Check sheet for the modelled part. Datum: model origin and axes. Units: mm. Round coordinates to 2 decimals unless told otherwise and drop trailing zeros. Loops run counter-clockwise (first coordinate to the right, second up) from the corner with the lowest first, then second, coordinate; pieces in that order, holes last. Notation, with made-up numbers: (69.25, -1.75) - (115.25, -1.75) arc R25 ccw to (115.25, 20.25) - close; hole circle Ø11 at (23.5, 8.25). An arc over 180 degrees is marked (long way). Put each result on its own line as item: value. Start each with the question number.
Item 1: Section check D-D, the plane x = 10.5. Record the cut outline in (y, z) (3 decimals), and give its area (3 significant figures).
Item 2: Material ranges on line 1 along X through (y, z) = (2.9, -32); line 2 along Z through (x, y) = (41, 0.5); line 3 along X through (y, z) = (1.55, 0), recorded low to high.
Item 3: Section check A-A, the plane x = -38.5. Record the cut outline in (y, z) (3 decimals).
Item 4: Section check C-C, the plane z = 0. Record the cut outline in (x, y) (3 decimals).
Item 5: Section check B-B, the plane y = 1. Record the cut outline in (x, z).
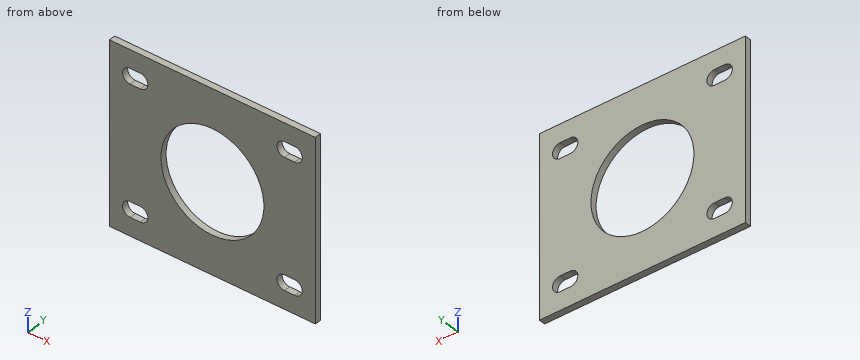
from build123d import *

# Parameters (mm, degrees)
SKETCH1_W           = 101.6
SKETCH1_H           = 88.9
SKETCH1_R           = 25.4
BOSS_EXTRUDE1_DEPTH = 3.175
CUT_EXTRUDE1_DEPTH  = 68.576054376


with BuildPart() as part:
    # Sketch1 → Boss-Extrude1 (new body)
    with BuildSketch(Plane(origin=(0, 0, 0), x_dir=(1, 0, 0), z_dir=(0, 1, 0))):
        Rectangle(SKETCH1_W, SKETCH1_H)
        with Locations(Location((0, 0, 0), (0, 0, 270))):
            Circle(SKETCH1_R, mode=Mode.SUBTRACT)
    extrude(amount=BOSS_EXTRUDE1_DEPTH)

    # Sketch2 → Cut-Extrude1 (cut, through all)
    with BuildSketch(Plane(origin=(0, 3.175, 0), x_dir=(1, 0, 0), z_dir=(0, 1, 0))):
        with BuildLine():
            Line((-40.6, 35.5), (-35.6, 35.5))
            ThreePointArc((-35.6, 35.5), (-31.85, 31.75), (-35.6, 28))
            Line((-35.6, 28), (-40.6, 28))
            ThreePointArc((-40.6, 28), (-44.35, 31.75), (-40.6, 35.5))
        make_face()
        with BuildLine():
            Line((-40.6, -28), (-35.6, -28))
            ThreePointArc((-35.6, -28), (-31.85, -31.75), (-35.6, -35.5))
            Line((-35.6, -35.5), (-40.6, -35.5))
            ThreePointArc((-40.6, -35.5), (-44.35, -31.75), (-40.6, -28))
        make_face()
        with BuildLine():
            Line((35.6, 35.5), (40.6, 35.5))
            ThreePointArc((40.6, 35.5), (44.35, 31.75), (40.6, 28))
            Line((40.6, 28), (35.6, 28))
            ThreePointArc((35.6, 28), (31.85, 31.75), (35.6, 35.5))
        make_face()
        with BuildLine():
            Line((35.6, -28), (40.6, -28))
            ThreePointArc((40.6, -28), (44.35, -31.75), (40.6, -35.5))
            Line((40.6, -35.5), (35.6, -35.5))
            ThreePointArc((35.6, -35.5), (31.85, -31.75), (35.6, -28))
        make_face()
    extrude(amount=-CUT_EXTRUDE1_DEPTH, mode=Mode.SUBTRACT)


solid = part.part
Check result:
1. outline: (0, -44.45) - (3.175, -44.45) - (3.175, -23.128) - (0, -23.128) - close; (0, 23.128) - (3.175, 23.128) - (3.175, 44.45) - (0, 44.45) - close
1. area: 135 mm²
2. line 1: -50.8 to -44.34, -31.86 to 31.86, 44.34 to 50.8
2. line 2: -44.45 to -35.48, -28.02 to 28.02, 35.48 to 44.45
2. line 3: -50.8 to -25.4, 25.4 to 50.8
3. outline: (0, -44.45) - (3.175, -44.45) - (3.175, -35.5) - (0, -35.5) - close; (0, -28) - (3.175, -28) - (3.175, 28) - (0, 28) - close; (0, 35.5) - (3.175, 35.5) - (3.175, 44.45) - (0, 44.45) - close
4. outline: (-50.8, 0) - (-25.4, 0) - (-25.4, 3.175) - (-50.8, 3.175) - close; (25.4, 0) - (50.8, 0) - (50.8, 3.175) - (25.4, 3.175) - close
5. outline: (-50.8, -44.45) - (50.8, -44.45) - (50.8, 44.45) - (-50.8, 44.45) - close; hole (-40.6, -35.5) - (-35.6, -35.5) arc R3.75 ccw to (-35.6, -28) - (-40.6, -28) arc R3.75 ccw to start; hole (-40.6, 28) - (-35.6, 28) arc R3.75 ccw to (-35.6, 35.5) - (-40.6, 35.5) arc R3.75 ccw to start; hole circle Ø50.8 at (0, 0); hole (35.6, -35.5) - (40.6, -35.5) arc R3.75 ccw to (40.6, -28) - (35.6, -28) arc R3.75 ccw to start; hole (35.6, 28) - (40.6, 28) arc R3.75 ccw to (40.6, 35.5) - (35.6, 35.5) arc R3.75 ccw to start
